Part model, mm, in its own coordinate system. Face numbers are marked on the shaded views. A direction names the side the tool comes from. Round coordinates to 2 decimals unless told otherwise and drop trailing zeros. Write each loop counter-clockwise with the first axis right and the second up, starting at its lowest first coordinate (ties: lowest second). Pieces come first, ordered by that corner, then holes. Notation, with made-up numbers: (6.25, 6.5) -> (50.25, 6.5) arc R14 cw to (50.25, 10.5) -> close; hole circle Ø2 at (41, -4). An arc over 180 degrees is marked (long way). Return JSON: item names as keys, results as strings. Group by question number.
(1) Drop flat-ended pins along their axis: pin 1 Ø4 at (x, z) = (107, 39) entering from -Y; pin 2 Ø10 at (y, z) = (40, 5) entering from +X; pin 3 Ø12 at (x, z) = (75, 7.5) entering from -Y (3 decimals). Give the stop position or say it passes through.
(2) Drill centre lines: L1, parallel to Y at x = 0, z = 16; L2, parallel to X at y = -26.5, z = -0.5; L3, parallel to Y at x = -9, z = -13.5. Where is each one in solid material? Low to high. Write a range as from..to.
(3) Tool access for the marked faces 4, 5 and 6: list every direction of +Z, -Z, +X, -X, +Y, -Y with a clear straight run to the whole face (end or side of a thin tool).
(4) Saw through at B-B (y = 34). List the corners of the cut face in (x, z).
(5) Saw through at A-A (x = 0). List the corners of the cut face in (y, z).
(6) Saw through at D-D (x = 143). List the corners of the cut face in (y, z), plus the area to 3 significant figures.
(7) Saw through at C-C (z = 29). List the corners of the cut face in (x, y), plus the area to 3 significant figures.
(8) Mould opens along X. For the marked faces 1, 2 and 3 say: +X half, -X half, draft (parallel to the pull), parting line (faces both ways), or undercut.
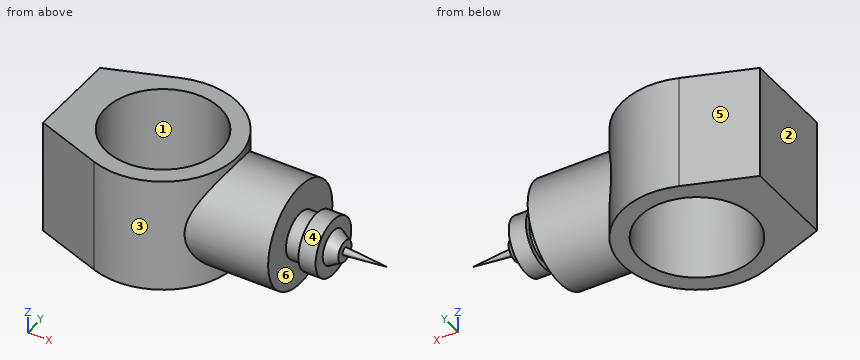
from build123d import *

# Parameters (mm, degrees)
CROQUIS1_R                   = 50
SALIENTE_EXTRUIR1_DEPTH      = 50
SALIENTE_EXTRUIR2_REACH      = 218.16
SALIENTE_EXTRUIR2_END_RADIUS = 65
CROQUIS2_R                   = 45


with BuildPart() as part:
    # Croquis1 → Saliente-Extruir1 (new, symmetric)
    with BuildSketch(Plane.XY):
        with BuildLine():
            Line((-80, -40), (-80, 40))
            Line((-80, 40), (-22.281665693, 61.061668614))
            ThreePointArc((-22.281665693, 61.061668614), (65, 0), (-22.281665693, -61.061668614))
            Line((-22.281665693, -61.061668614), (-80, -40))
        make_face()
        Circle(CROQUIS1_R, mode=Mode.SUBTRACT)
    extrude(amount=SALIENTE_EXTRUIR1_DEPTH, both=True)

    # Saliente-Extruir2: up to this cylinder (the profile starts outside it)
    saliente_extruir2_end = Plane(origin=(0, 0, 0), z_dir=(0, 0, -1)) * Cylinder(SALIENTE_EXTRUIR2_END_RADIUS, 567.32, mode=Mode.PRIVATE)
    # Croquis2 → Saliente-Extruir2 (add, up to the surface)
    with BuildSketch(Plane(origin=(120, 0, 0), x_dir=(0, 0, -1), z_dir=(1, 0, 0)), mode=Mode.PRIVATE) as saliente_extruir2_sk1:
        Circle(CROQUIS2_R)
    saliente_extruir2_tool1 = extrude(saliente_extruir2_sk1.sketch, amount=-SALIENTE_EXTRUIR2_REACH, mode=Mode.PRIVATE) - saliente_extruir2_end
    add(saliente_extruir2_tool1.solids().sort_by_distance((120, 0, 0))[0])

    # Croquis3 → Revolución1 (revolve)
    with BuildSketch(Plane.XY, mode=Mode.PRIVATE) as revoluci_n1_sk:
        Polygon((120, 0), (120, -20), (134, -20), (134, -25), (149, -25), (149, -15), (159, -9.215277891), (159, -3.215277891), (195.860032394, 0), align=None)
    revolve(revoluci_n1_sk.sketch.rotate(Axis((0, 0, 0), (1, 0, 0)), 270), axis=Axis((0, 0, 0), (1, 0, 0)))


solid = part.part
Computed values:
{
 "1": {"pin 1": "y = -25.61", "pin 2": "x = 120", "pin 3": "y = -44.975"},
 "2": {"L1": "-65..-50, 50..65", "L2": "-80..-42.4, 42.4..120", "L3": "-64.37..-49.18, 49.18..64.37"},
 "3": {"face 4": "+X", "face 5": "+Z, -Z, -X, +Y", "face 6": "none"},
 "4": {"outline": "(-80, -50) -> (-36.66, -50) -> (-36.66, 50) -> (-80, 50) -> close; (36.66, -50) -> (55.4, -50) -> (55.4, -29.48) -> (120, -29.48) -> (120, 29.48) -> (55.4, 29.48) -> (55.4, 50) -> (36.66, 50) -> close"},
 "5": {"outline": "(-65, -50) -> (-50, -50) -> (-50, 50) -> (-65, 50) -> close; (50, -50) -> (65, -50) -> (65, 50) -> (50, 50) -> close"},
 "6": {"outline": "circle Ø50 at (0, 0)", "area": "1,960 mm2"},
 "7": {"outline": "(-80, -40) -> (-22.28, -61.06) arc R65 ccw to (55.15, -34.41) -> (120, -34.41) -> (120, 34.41) -> (55.15, 34.41) arc R65 ccw to (-22.28, 61.06) -> (-80, 40) -> close; hole circle Ø100 at (0, 0)", "area": "11,500 mm2"},
 "8": {"face 1": "undercut", "face 2": "-X half", "face 3": "parting line"}
}
